The model under review builds one solid part; all positions refer to its coordinate system, in mm. A direction names the side the tool comes from. Round coordinates to 2 decimals unless told otherwise and drop trailing zeros. Write each loop counter-clockwise with the first axis right and the second up, starting at its lowest first coordinate (ties: lowest second). Pieces come first, ordered by that corner, then holes. Notation, with made-up numbers: (85.25, 27) - (105.25, 27) arc R18 cw to (105.25, 34) - close; hole circle Ø2 at (34.25, 28). An arc over 180 degrees is marked (long way). Return JSON: item names as keys, results as strings.
from build123d import *

# Parameters (mm, degrees)
SKETCH1_W           = 129
SKETCH1_H           = 129
SKETCH1_W_2         = 69
SKETCH1_H_2         = 69
EXTRUDE_THIN1_DEPTH = 10
EXTRUDE_THIN1_DRAFT = 14
FILLET1_R           = 10
SKETCH3_W           = 129
SKETCH3_H           = 129
BOSS_EXTRUDE1_DEPTH = 2
SKETCH4_R           = 2.5
CUT_EXTRUDE1_DEPTH  = 2
SKETCH5_W           = 129
SKETCH5_H           = 129
SKETCH5_W_2         = 119
SKETCH5_H_2         = 119
EXTRUDE_THIN2_DEPTH = 30
CUT_EXTRUDE2_DEPTH  = 5
SKETCH7_R           = 2.5
CUT_EXTRUDE3_DEPTH  = 12
FILLET2_R           = 10
SKETCH8_W           = 79
SKETCH8_H           = 5
CUT_EXTRUDE4_DEPTH  = 5
SKETCH9_R           = 8
CUT_EXTRUDE5_DEPTH  = 12
SKETCH9_3_R         = 8
CUT_EXTRUDE6_DEPTH  = 12


with BuildPart() as part:
    # Sketch1 → Extrude-Thin1 (with draft: the straight prism first)
    with BuildSketch(Plane(origin=(0, 0, 0), x_dir=(1, 0, 0), z_dir=(0, 1, 0))):
        Rectangle(SKETCH1_W, SKETCH1_H)
        Rectangle(SKETCH1_W_2, SKETCH1_H_2, mode=Mode.SUBTRACT)
    extrude(amount=EXTRUDE_THIN1_DEPTH)
    # Extrude-Thin1: the draft: its side faces are tilted about the plane it starts from
    extrude_thin1_sides = [part.faces().sort_by_distance(p)[0] for p in [
        (0, 5, -64.5),
        (-64.5, 5, 0),
        (0, 5, 64.5),
        (64.5, 5, 0),
        (34.5, 5, 0),
        (0, 5, 34.5),
        (-34.5, 5, 0),
        (0, 5, -34.5),
    ]]
    draft(extrude_thin1_sides, Plane(origin=(0, 0, 0), x_dir=(1, 0, 0), z_dir=(0, 1, 0)), EXTRUDE_THIN1_DRAFT)

    # Fillet1
    fillet1_edges = [part.edges().sort_by_distance(p)[0] for p in [
        (35.746640014, 5, 35.746640014),
        (35.746640014, 5, -35.746640014),
        (-35.746640014, 5, -35.746640014),
        (-35.746640014, 5, 35.746640014),
    ]]
    fillet(fillet1_edges, radius=FILLET1_R)

    # Sketch3 → Boss-Extrude1 (add)
    with BuildSketch(Plane.XZ):
        Rectangle(SKETCH3_W, SKETCH3_H)
    extrude(amount=BOSS_EXTRUDE1_DEPTH)

    # Sketch4 → Cut-Extrude1 (cut)
    with BuildSketch(Plane(origin=(0, 0, 0), x_dir=(1, 0, 0), z_dir=(0, 1, 0))):
        with Locations(Location((-22.5, 0, 0), (0, 0, 270))):
            Circle(SKETCH4_R)
    cut_extrude1 = extrude(amount=-CUT_EXTRUDE1_DEPTH, mode=Mode.SUBTRACT)

    # Mirror1: Cut-Extrude1 across plane
    add(cut_extrude1.mirror(Plane(origin=(0, 0, 0), x_dir=(0, 0, 1), z_dir=(1, 0, 0))), mode=Mode.SUBTRACT)

    # Sketch5 → Extrude-Thin2 (add)
    with BuildSketch(Plane.XZ.offset(2)):
        Rectangle(SKETCH5_W, SKETCH5_H)
        Rectangle(SKETCH5_W_2, SKETCH5_H_2, mode=Mode.SUBTRACT)
    extrude(amount=EXTRUDE_THIN2_DEPTH)

    # Sketch6 → Cut-Extrude2 (cut)
    with BuildSketch(Plane.XY.offset(64.5)):
        with BuildLine():
            Line((-5, -32), (5, -32))
            ThreePointArc((5, -32), (0, -27), (-5, -32))
        make_face()
    extrude(amount=-CUT_EXTRUDE2_DEPTH, mode=Mode.SUBTRACT)

    # Sketch7 → Cut-Extrude3 (cut)
    with BuildSketch(Plane(origin=(0, 10, 0), x_dir=(1, 0, 0), z_dir=(0, 1, 0))):
        with Locations(Location((0, -40.493280028, 0), (0, 0, 270))):
            Circle(SKETCH7_R)
    extrude(amount=-CUT_EXTRUDE3_DEPTH, mode=Mode.SUBTRACT)

    # Fillet2
    # the kernel refuses this fillet: 10 mm, written as the material it takes off along each edge
    with BuildSketch(Plane(origin=(-64.5, -57, -64.5), x_dir=(1, 0, 0), z_dir=(0, 1, 0)), Plane(origin=(64.5, 25, -64.5), x_dir=(-1, 0, 0), z_dir=(0, -1, 0)), Plane(origin=(-64.5, -57, 64.5), x_dir=(0, 0, -1), z_dir=(0, 1, 0))) as fillet2_piece_1:
        with BuildLine():
            CenterArc((FILLET2_R, -FILLET2_R), FILLET2_R, 90, 90)
            Line((0, -FILLET2_R), (0, 0))
            Line((0, 0), (FILLET2_R, 0))
        make_face()
    extrude(amount=82, mode=Mode.SUBTRACT)
    with BuildSketch(Plane(origin=(64.5, -57, 64.5), x_dir=(0, 0, -1), z_dir=(0, 1, 0))) as fillet2_piece_2:
        with BuildLine():
            CenterArc((FILLET2_R, FILLET2_R), FILLET2_R, 180, 90)
            Line((0, FILLET2_R), (0, 0))
            Line((0, 0), (FILLET2_R, 0))
        make_face()
    extrude(amount=82, mode=Mode.SUBTRACT)
    with BuildSketch(Plane(origin=(70.043929395, -22.235486312, 70.043929395), x_dir=(0.05688523373566075, -0.22815421086671833, -0.9719617925858115), z_dir=(-0.23513883931281052, 0.9430903734495696, -0.23513883931281052)), Plane(origin=(70.043929395, -22.235486312, -70.043929395), x_dir=(-0.9719617925858115, -0.22815421086671833, -0.05688523373566075), z_dir=(-0.23513883931281052, 0.9430903734495696, 0.23513883931281052))) as fillet2_piece_3:
        with BuildLine():
            CenterArc((FILLET2_R * 0.94309037345, FILLET2_R), FILLET2_R, 183.355221767, 86.644778233)
            Line((-FILLET2_R * 0.0551954991819, FILLET2_R * 0.941473796429), (0, 0))
            Line((0, 0), (FILLET2_R * 0.94309037345, 0))
        make_face()
    extrude(amount=57.757956351, mode=Mode.SUBTRACT)
    with BuildSketch(Plane(origin=(-70.043929395, -22.235486312, 70.043929395), x_dir=(-0.05688523373566065, -0.22815421086671833, -0.9719617925858115), z_dir=(0.23513883931281052, 0.9430903734495696, -0.23513883931281052)), Plane(origin=(-70.043929395, -22.235486312, -70.043929395), x_dir=(0.9719617925858115, -0.22815421086671833, -0.05688523373566065), z_dir=(0.23513883931281052, 0.9430903734495696, 0.23513883931281052))) as fillet2_piece_4:
        with BuildLine():
            CenterArc((FILLET2_R * 0.94309037345, -FILLET2_R), FILLET2_R, 90, 86.644778233)
            Line((-FILLET2_R * 0.0551954991819, -FILLET2_R * 0.941473796429), (0, 0))
            Line((0, 0), (FILLET2_R * 0.94309037345, 0))
        make_face()
    extrude(amount=57.757956351, mode=Mode.SUBTRACT)

    # Sketch8 → Cut-Extrude4 (cut)
    with BuildSketch(Plane(origin=(0, 0, -64.5), x_dir=(-1, 0, 0), z_dir=(0, 0, -1))):
        with Locations((0, -19.5)):
            Rectangle(SKETCH8_W, SKETCH8_H)
    extrude(amount=-CUT_EXTRUDE4_DEPTH, mode=Mode.SUBTRACT)

    # Sketch9 → Cut-Extrude5 (cut)
    with BuildSketch(Plane(origin=(0, 10, 0), x_dir=(1, 0, 0), z_dir=(0, 1, 0))):
        with Locations(Location((49.006719972, 49.5, 0), (0, 0, 270))):
            Circle(SKETCH9_R)
    extrude(amount=-CUT_EXTRUDE5_DEPTH, mode=Mode.SUBTRACT)

    # Sketch9<3> → Cut-Extrude6 (cut)
    with BuildSketch(Plane(origin=(0, 10, 0), x_dir=(1, 0, 0), z_dir=(0, 1, 0))):
        with Locations(Location((49.006719972, 49.5, 0), (0, 0, 270))):
            Circle(SKETCH9_3_R)
        with Locations(Location((24.006719972, 49.5, 0), (0, 0, 270))):
            Circle(SKETCH9_3_R)
    extrude(amount=-CUT_EXTRUDE6_DEPTH, mode=Mode.SUBTRACT)


solid = part.part
(1) Wall thickness on line 1 (Z direction, x = 47.5, y = -20); line 2 (X direction, y = -1.1, z = 0): over which ranges is each line inside the solid? List them lowest first.
Filled in:
{"line 1": "z = -64.5 to -59.5, 59.5 to 64.5", "line 2": "x = -64.5 to -25, -20 to 20, 25 to 64.5"}
(2) Add section D-D (x = 22.5). Write out the cut boundary in (y, z).
Filled in:
{"outline": "(-32, -64.5) - (-22, -64.5) - (-22, -59.5) - (-32, -59.5) - close; (-32, 59.5) - (-2, 59.5) - (-2, 2.5) - (0, 2.5) - (0, 34.5) - (10, 36.99) - (10, 62.01) - (0, 64.5) - (-32, 64.5) - close; (-17, -64.5) - (0, -64.5) - (10, -62.01) - (10, -57.36) - (-2, -57.36) - (-2, -59.5) - (-17, -59.5) - close; (-2, -41.64) - (10, -41.64) - (10, -36.99) - (0, -34.5) - (0, -2.5) - (-2, -2.5) - close"}
(3) Add section A-A (x = 0). Write out the cut boundary in (y, z), plus the area to 3 significant figures.
Filled in:
{"outline": "(-32, -64.5) - (-22, -64.5) - (-22, -59.5) - (-32, -59.5) - close; (-27, 59.5) - (-2, 59.5) - (-2, 42.99) - (10, 42.99) - (10, 62.01) - (0, 64.5) - (-27, 64.5) - close; (-17, -64.5) - (0, -64.5) - (10, -62.01) - (10, -36.99) - (0, -34.5) - (0, 34.5) - (10, 36.99) - (10, 37.99) - (-2, 37.99) - (-2, -59.5) - (-17, -59.5) - close", "area": "998 mm2"}
(4) Clearance check with flat-ended pins moving along their axes: pin 1 Ø6 at (x, z) = (0, 40.49) entering from -Y; pin 2 Ø3 at (y, z) = (4, 17) entering from +X; pin 3 Ø8 at (x, z) = (22.5, 0) entering from +Y. State where each tip first meets the part, or that it passes through.
Filled in:
{"pin 1": "stops at y = -2", "pin 2": "stops at x = 63.88", "pin 3": "stops at y = 0"}
(5) Add section B-B (z = -49.5). Write out the cut boundary in (x, y), plus the area to 3 significant figures.
Filled in:
{"outline": "(-64.5, -32) - (-59.5, -32) - (-59.5, -2) - (16.01, -2) - (16.01, 10) - (-62.01, 10) - (-64.5, 0) - close; (32.01, -2) - (41.01, -2) - (41.01, 10) - (32.01, 10) - close; (57.01, -2) - (59.5, -2) - (59.5, -32) - (64.5, -32) - (64.5, 0) - (62.01, 10) - (57.01, 10) - close", "area": "1,440 mm2"}
(6) Add section C-C (y = -4.5). Write out the cut boundary in (x, z).
Filled in:
{"outline": "(-64.5, -54.5) arc R10 ccw to (-54.5, -64.5) - (54.5, -64.5) arc R10 ccw to (64.5, -54.5) - (64.5, 54.5) arc R10 ccw to (54.5, 64.5) - (-54.5, 64.5) arc R10 ccw to (-64.5, 54.5) - close; hole (-59.5, -59.5) - (59.5, -59.5) - (59.5, 59.5) - (-59.5, 59.5) - close"}
(7) Mouldability with a two-part tool opening along X and no side actions: class faces 1 (the flat face through (64.5, -16, -1)), 2 (the flat face through (59.5, -17, -1)), 3 (the cylindrical face through (-60.223, 5.587, -60.373)), 4 (the flat face through (-1, -17, 59.5)) as released by +X, released by -X, zero draft, split by the parting line, or undercut.
Filled in:
{"face 1": "released by +X", "face 2": "undercut", "face 3": "released by -X", "face 4": "undercut"}
(8) For faces 5 (the cylindrical face through (-32.794, 4.725, -32.944)), 6 (the cylindrical face through (0, -27, 62)), 7 (the flat face through (39.5, -20, -62)), 8 (the cylindrical face through (-20, -1, 0)), 9 (the flat face through (-59.5, -17, -1)), list the 3-axis set-ups (+Z, -Z, +X, -X, +Y, -Y) from which the entire face can be reached by the end or side of a thin tool; tool diameter is ignored.
Filled in:
{"face 5": "+Y", "face 6": "+Z, -Y", "face 7": "-Z", "face 8": "+Y, -Y", "face 9": "-Y"}
